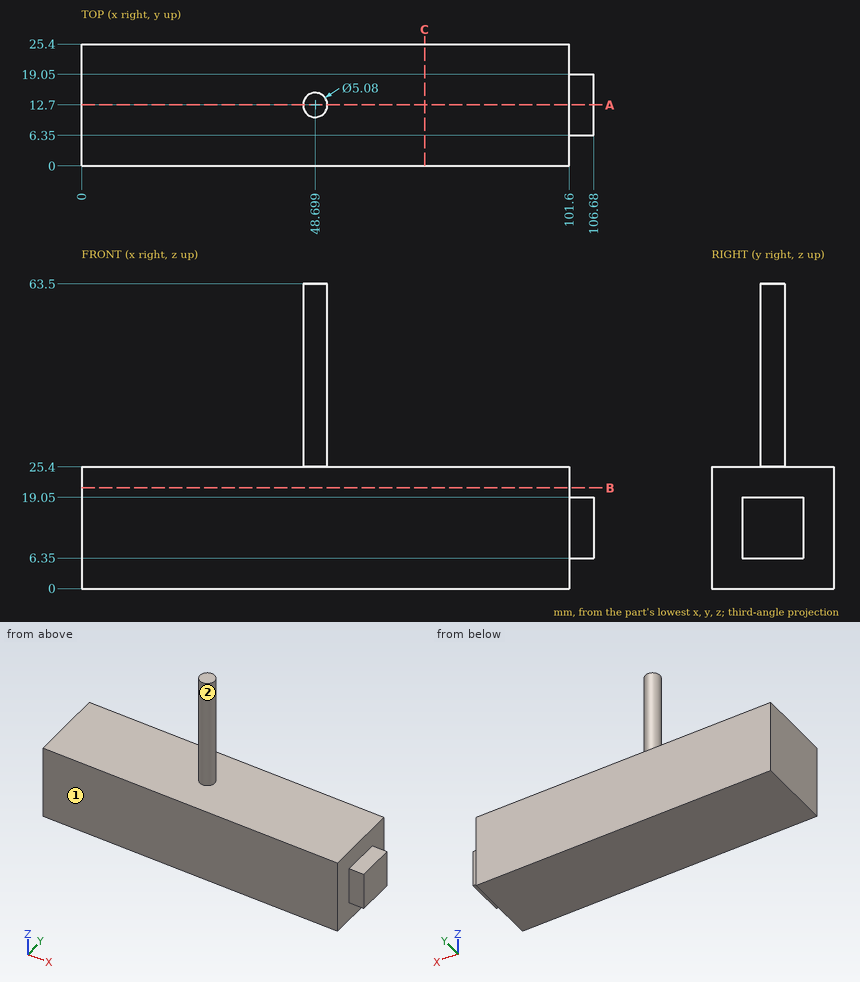
Geometry check sheet. Reference: drawing and pictorial views, mm from the part's lowest x, y, z. A direction names the side the tool comes from. Coordinates: 2 decimals unless noted, no trailing zeros. Write each loop counter-clockwise with the first axis right and the second up, starting at its lowest first coordinate (ties: lowest second). Pieces come first, ordered by that corner, then holes. Notation, with made-up numbers: (3.25, 18.25) - (54.25, 18.25) arc R15 cw to (54.25, 29.25) - close; hole circle Ø3 at (48.5, 63.5). An arc over 180 degrees is marked (long way). One line per question, with ' | ' between items. Start each with the question number.
1. Section check B-B (z = 21). Enter the section's corners in (x, y), plus the area to 3 significant figures.
2. Gauge pin test, flat ends, axial feed: P1, Ø4, axis at x = 104, y = 10, coming from the +Z side; P2, Ø1.5, axis at x = 14, z = 28, coming from the +Y side; P3, Ø1.5, axis at x = 104, z = 10.5, coming from the +Y side; P4, Ø1.5, axis at x = 103.5, y = 12.5, coming from the -Z side. Record the tip position at first contact, or that the pin passes through.
3. Material ranges on line 1 along X through (y, z) = (16.5, 4.5); line 2 along Z through (x, y) = (15, 16); line 3 along Y through (x, z) = (48, 59), recorded low to high.
4. Access from +Z, -Z, +X, -X, +Y, -Y to the whole of each face (thin tool, end or side, straight path). Record for the marked faces 1 and 2.
5. Section check C-C (x = 71.5). Enter the section's corners in (y, z), plus the area to 3 significant figures.
6. Section check A-A (y = 12.7). Enter the section's corners in (x, z).
Computed values:
1) outline: (0, 0) - (101.6, 0) - (101.6, 25.4) - (0, 25.4) - close | area: 2,580 mm²
2) P1: z = 19.05 | P2: through | P3: y = 19.05 | P4: z = 6.35
3) line 1: 0 to 101.6 | line 2: 0 to 25.4 | line 3: 10.26 to 15.14
4) face 1: +Z, -Z, +X, -X, -Y | face 2: +Z
5) outline: (0, 0) - (25.4, 0) - (25.4, 25.4) - (0, 25.4) - close | area: 645 mm²
6) outline: (0, 0) - (101.6, 0) - (101.6, 6.35) - (106.68, 6.35) - (106.68, 19.05) - (101.6, 19.05) - (101.6, 25.4) - (51.24, 25.4) - (51.24, 63.5) - (46.16, 63.5) - (46.16, 25.4) - (0, 25.4) - close
